from build123d import *

# Parameters (mm, degrees)
SKETCH1_W           = 6.35
SKETCH1_H           = 66.675
BOSS_EXTRUDE1_DEPTH = 15.875
SKETCH2_R           = 15.875
BOSS_EXTRUDE2_DEPTH = 31.75
SKETCH3_R           = 20.955
BOSS_EXTRUDE3_DEPTH = 9.525


with BuildPart() as part:
    # Sketch1 → Boss-Extrude1 (new, symmetric)
    with BuildSketch(Plane.XY):
        with Locations((3.175, -33.3375)):
            Rectangle(SKETCH1_W, SKETCH1_H)
    extrude(amount=BOSS_EXTRUDE1_DEPTH, both=True)

    # Sketch2 → Boss-Extrude2 (add)
    with BuildSketch(Plane.ZY):
        with Locations(Location((0, 0, 0), (0, 0, 270))):
            Circle(SKETCH2_R)
    extrude(amount=-BOSS_EXTRUDE2_DEPTH)

    # Sketch3 → Boss-Extrude3 (add)
    with BuildSketch(Plane.ZY):
        with Locations(Location((0, 0, 0), (0, 0, 220.749054377))):
            Circle(SKETCH3_R)
    extrude(amount=BOSS_EXTRUDE3_DEPTH)

    # Sketch4 → Cut-Revolve1 (revolve, cut)
    with BuildSketch(Plane.XY):
        Polygon((-9.525, 19.1135), (-6.35, 19.1135), (-6.35, 9.652), (31.75, 9.652), (31.75, 0), (-9.525, 0), align=None)
    revolve(axis=Axis((31.75, 0, 0), (-1, 0, 0)), mode=Mode.SUBTRACT)


solid = part.part
Build history of the part. All positions in model axes, mm. A direction names the side the tool comes from. Round coordinates to 2 decimals unless told otherwise and drop trailing zeros. Write each loop counter-clockwise with the first axis right and the second up, starting at its lowest first coordinate (ties: lowest second). Pieces come first, ordered by that corner, then holes. Notation, with made-up numbers: M 67.5,-16 L 81.5,-16 A22 cw 81.5,22 Z; hole C -36.75,-11 d1. An arc over 180 degrees is marked long. Answer as a JSON object with one key per item and string values. Group by question number.
(1) Cut at B-B (y = 4.5). Give the cut face in (x, z) (3 decimals).
(2) Cut at D-D (z = -11.5). Give the cut face in (x, y) (3 decimals), and give its area (3 significant figures).
(3) Drill centre lines: L1, parallel to Z at x = -8.4, y = 0 (1 decimal); L2, parallel to Z at x = 13, y = 0 (3 decimals). Where is each one in solid material? Low to high.
(4) Flat gauge pins, fed straight in: pin 1 (1.5 mm diameter, centred on x = 3.5, y = -35, fed in from +Z) (3 decimals); pin 2 (10 mm diameter, centred on y = -29, z = -10, fed in from -X); pin 3 (6 mm diameter, centred on x = 27, z = 4.5, fed in from -Y). Where does each tip first touch, or does it go through?
(5) Cut at C-C (x = 15.5). Give the cut face in (y, z) (3 decimals), and give its area (3 significant figures).
(6) Which spindle directions (+Z, -Z, +X, -X, +Y, -Y) get a long thin tool onto all of the face, cutting with end or side? Do faces 1 (the flat face through (3, -33, 15.875)), 2 (the flat face through (-6.35, -9, -5)), 3 (the flat face through (3, -33, -15.875)), 4 (the flat face through (0, 15, 6)). Say none if no direction does.
Responses:
{
 "1": {"outline": "M -9.525,-20.466 L 0,-20.466 L 0,-15.224 L 31.75,-15.224 L 31.75,-8.539 L -6.35,-8.539 L -6.35,-18.576 L -9.525,-18.576 Z; M -9.525,18.576 L -6.35,18.576 L -6.35,8.539 L 31.75,8.539 L 31.75,15.224 L 0,15.224 L 0,20.466 L -9.525,20.466 Z"},
 "2": {"outline": "M -9.525,-17.517 L 0,-17.517 L 0,-66.675 L 6.35,-66.675 L 6.35,-10.944 L 31.75,-10.944 L 31.75,10.944 L 0,10.944 L 0,17.517 L -9.525,17.517 L -9.525,15.267 L -6.35,15.267 L -6.35,-15.267 L -9.525,-15.267 Z", "area": "1,290 mm2"},
 "3": {"L1": "z = -21 to -19.1, 19.1 to 21", "L2": "z = -15.875 to -9.652, 9.652 to 15.875"},
 "4": {"pin 1": "stops at z = 15.875", "pin 2": "stops at x = 0", "pin 3": "stops at y = -15.8"},
 "5": {"outline": "C 0,0 d31.75; hole C 0,0 d19.304", "area": "499 mm2"},
 "6": {"face 1": "+Z, +X, +Y, -Y", "face 2": "-X", "face 3": "-Z, +X, +Y, -Y", "face 4": "+X, +Y"}
}
